Input: part model. Units: mm. Frame: model coordinates. Give positions to 0.01 mm unless a question says otherwise; leave off trailing zeros. Write each loop counter-clockwise with the first axis right and the second up, starting at its lowest first coordinate (ties: lowest second). Pieces come first, ordered by that corner, then holes. Notation, with made-up numbers: (29, 40.5) - (55, 40.5) arc R16 ccw to (55, 45.5) - close; hole circle Ø11 at (-11.75, 64). An arc over 180 degrees is marked (long way). Answer as a JSON object with one key per item and string values. Group by question number.
from build123d import *

# Parameters (mm, degrees)
SKETCH3_W                    = 914.4
SKETCH3_H                    = 609.6
BOSS_EXTRUDE1_DEPTH          = 0.79375
SKETCH4_OUTSIDE_W            = 1136.194
SKETCH4_OUTSIDE_H            = 831.394
CUT_EXTRUDE1_DEPTH           = 2.54
CUT_EXTRUDE2_DEPTH           = 2.54
CUT_EXTRUDE3_DEPTH           = 2.54
F_10_0_1935_DIAMETER_HOLE1_D = 4.9149
F_10_0_1935_DIAMETER_HOLE2_D = 4.9149


with BuildPart() as part:
    # Sketch3 → Boss-Extrude1 (new, symmetric)
    with BuildSketch(Plane.XY):
        Rectangle(SKETCH3_W, SKETCH3_H)
    extrude(amount=BOSS_EXTRUDE1_DEPTH, both=True)

    # Sketch4 outside → Cut-Extrude1 (cut)
    with BuildSketch(Plane.XY.offset(0.79375)):
        Rectangle(SKETCH4_OUTSIDE_W, SKETCH4_OUTSIDE_H)
        with BuildLine():
            Line((-352.134938229, -305.170644008), (-377.534938229, -279.770644008))
            Line((-377.534938229, -279.770644008), (-377.534938229, -42.598144008))
            ThreePointArc((-377.534938229, -42.598144008), (-376.790989453, -40.802092784), (-374.994938229, -40.058144008))
            Line((-374.994938229, -40.058144008), (331.125061771, -40.058144008))
            ThreePointArc((331.125061771, -40.058144008), (332.921112995, -40.802092784), (333.665061771, -42.598144008))
            Line((333.665061771, -42.598144008), (333.665061771, -279.770644008))
            Line((333.665061771, -279.770644008), (308.265061771, -305.170644008))
            Line((308.265061771, -305.170644008), (-352.134938229, -305.170644008))
        make_face(mode=Mode.SUBTRACT)
    extrude(amount=-CUT_EXTRUDE1_DEPTH, mode=Mode.SUBTRACT)

    # Sketch7 → Cut-Extrude2 (cut)
    with BuildSketch(Plane.XY.offset(0.79375)):
        with BuildLine():
            Line((-377.534938229, -188.190344021), (-377.534938229, -40.058144008))
            Line((-377.534938229, -40.058144008), (-229.402738216, -40.058144008))
            Line((-229.402738216, -40.058144008), (-229.402738216, -64.746344021))
            Line((-229.402738216, -64.746344021), (-229.402738216, -121.896344021))
            ThreePointArc((-229.402738216, -121.896344021), (-248.819801264, -168.773280973), (-295.696738216, -188.190344021))
            Line((-295.696738216, -188.190344021), (-352.846738216, -188.190344021))
            Line((-352.846738216, -188.190344021), (-377.534938229, -188.190344021))
        make_face()
    extrude(amount=-CUT_EXTRUDE2_DEPTH, mode=Mode.SUBTRACT)

    # Sketch8 → Cut-Extrude3 (cut)
    with BuildSketch(Plane.XY.offset(0.79375)):
        with BuildLine():
            Line((251.115061771, -188.190344021), (336.840061771, -188.190344021))
            Line((336.840061771, -188.190344021), (336.840061771, -36.171344021))
            Line((336.840061771, -36.171344021), (184.821061771, -36.171344021))
            Line((184.821061771, -36.171344021), (184.821061771, -121.896344021))
            ThreePointArc((184.821061771, -121.896344021), (204.238124819, -168.773280973), (251.115061771, -188.190344021))
        make_face()
    extrude(amount=-CUT_EXTRUDE3_DEPTH, mode=Mode.SUBTRACT)

    # #10 (0.1935) Diameter Hole1 (through all)
    with Locations(Plane.XY.offset(0.79375)):
        with Locations((-314.034938229, -292.470644008), (-339.434938229, -292.470644008), (-364.834938229, -279.770644008), (86.005546883, -293.702239208), (111.405546883, -293.702239208), (214.149530262, -292.114748821), (239.549530262, -292.114748821), (296.276261771, -292.470644008), (270.876261771, -292.470644008), (321.676261771, -279.770644008), (174.915061771, -52.758144008), (-218.784938229, -52.758144008), (-72.379338229, -292.470644008), (29.220661771, -292.470644008)):
            Hole(F_10_0_1935_DIAMETER_HOLE1_D / 2)

    # #10 (0.1935) Diameter Hole2 (through all)
    with Locations(Plane.XY.offset(0.79375)):
        with Locations((-129.88493833, -121.629072033), (-129.88493833, -222.541034234), (86.015061873, -223.229071976), (86.015061873, -121.629072033)):
            Hole(F_10_0_1935_DIAMETER_HOLE2_D / 2)


solid = part.part
1) Cut plane C-C on x = -264.5. Return the cut outline in (y, z), and give its area (3 significant figures).
2) Cut plane A-A on z = -0.2. Count the separate pieces of the cut face and the enclosed holes in it, and give its area (3 significant figures).
3) Cut plane B-B on y = -72. Return the cut outline in (x, z), and give its area (3 significant figures).
4) Line query: line 1 along Y through (x, z) = (30, -0.6); line 2 along Y through (x, z) = (-333, 0.65); line 3 along X through (y, z) = (-224, -0.45). Output: solid intervals per line, ascending. Write a range as from..to.
5) Pin query (flat end, axial travel): P1, Ø0.5, axis at x = -329, z = 0.5, coming from the +Y side; P2, Ø4, axis at x = 296.28, y = -292.47, coming from the -Z side. Return the tip coordinate at first contact, or that it passes through.
Filled in:
{
 "1": {"outline": "(-304.8, -0.79) - (-180.39, -0.79) - (-180.39, 0.79) - (-304.8, 0.79) - close", "area": "197 mm²"},
 "2": {"separate pieces": "1", "enclosed holes": "18", "area": "145,000 mm²"},
 "3": {"outline": "(-229.4, -0.79) - (184.82, -0.79) - (184.82, 0.79) - (-229.4, 0.79) - close", "area": "658 mm²"},
 "4": {"line 1": "y = -304.8..-294.8, -290.14..-40.06", "line 2": "y = -304.8..-188.19", "line 3": "x = -377.53..-131.86, -127.91..83.68, 88.35..333.67"},
 "5": {"P1": "stops at y = -188.19", "P2": "passes through"}
}
